Part model, mm, in its own coordinate system. A direction names the side the tool comes from. Round coordinates to 2 decimals unless told otherwise and drop trailing zeros. Order: outer loops, then holes, each group sorted by start corner. A loop starts at its lowest first (then second) coordinate and runs counter-clockwise, first axis right, second up. Notation, with made-up numbers: (47, 40) - (55, 40) arc R17 ccw to (55, 70) - close; hole circle Ø10 at (-8, -37.5). An arc over 180 degrees is marked (long way). Return JSON: item names as keys, results as strings. Group by question number.
Item 1: Two-plate mould, pull along X, no slides. Class faces 3 (the face through (8, 55, -2)), 4 (the face through (3, 6, -7)), 5 (the face through (15, 20, -3)): released by +X, released by -X, zero draft, split by the parting line, or undercut.
Item 2: Saw through at B-B on z = -9. List the corners of the cut face in (x, y), and give its area (3 significant figures).
Item 3: Saw through at C-C on y = 37. List the corners of the cut face in (x, z), and give its area (3 significant figures).
Item 4: Saw through at A-A on x = 7.5. List the corners of the cut face in (y, z).
Item 5: Drop flat-ended pins along their axis: pin 1 (1 mm diameter, centred on x = 11.5, y = 14.5, fed in from -Z); pin 2 (6 mm diameter, centred on x = 4, z = -11.5, fed in from +Y). Give the stop position or say it passes through.
Item 6: Probe probe 1 along Z at (x, y) = (13.25, 39); probe 2 along X at (y, z) = (2.35, -9); probe 3 along Y at (x, z) = (6.5, -6.5). List the from-to ranges inside material, lowest first.
Item 7: Tool access for faces 1 (the face through (5, 3, -11)), 2 (the face through (7, 1, -15)): list every direction of +Z, -Z, +X, -X, +Y, -Y with a clear straight run to the whole face (end or side of a thin tool).
Item 8: Saw through at D-D on x = 11.25. List the corners of the cut face in (y, z).
```python
from build123d import *

# Parameters (mm, degrees)
SKETCH1_W           = 15
SKETCH1_H           = 15
SKETCH1_R           = 2.65
BOSS_EXTRUDE1_DEPTH = 3
SKETCH2_W           = 15
SKETCH2_H           = 4
BOSS_EXTRUDE2_DEPTH = 54
BOSS_EXTRUDE3_DEPTH = 3
SKETCH4_R           = 1.65
CUT_EXTRUDE1_DEPTH  = 13
CUT_EXTRUDE2_DEPTH  = 20


with BuildPart() as part:
    # Sketch1 → Boss-Extrude1 (new body)
    with BuildSketch(Plane(origin=(0, 0, 0), x_dir=(1, 0, 0), z_dir=(0, 1, 0))):
        with Locations((7.5, 7.5)):
            Rectangle(SKETCH1_W, SKETCH1_H)
        with Locations(Location((7.5, 9, 0), (0, 0, 270))):
            Circle(SKETCH1_R, mode=Mode.SUBTRACT)
    extrude(amount=BOSS_EXTRUDE1_DEPTH)

    # Sketch2 → Boss-Extrude2 (add)
    with BuildSketch(Plane(origin=(0, 3, 0), x_dir=(1, 0, 0), z_dir=(0, 1, 0))):
        with Locations((7.5, 2)):
            Rectangle(SKETCH2_W, SKETCH2_H)
    extrude(amount=BOSS_EXTRUDE2_DEPTH)

    # Sketch3 → Boss-Extrude3 (add)
    with BuildSketch(Plane(origin=(15, 0, 0), x_dir=(0, 0, -1), z_dir=(1, 0, 0))):
        Polygon((4, 14), (15, 3), (4, 3), align=None)
    boss_extrude3 = extrude(amount=-BOSS_EXTRUDE3_DEPTH)

    # Mirror1: Boss-Extrude3 across plane
    add(boss_extrude3.mirror(Plane.ZY.offset(-7.5)))

    # Sketch4 → Cut-Extrude1 (cut)
    with BuildSketch(Plane(origin=(0, 0, -4), x_dir=(-1, 0, 0), z_dir=(0, 0, -1))):
        with Locations((-7.5, 37)):
            Circle(SKETCH4_R)
    extrude(amount=-CUT_EXTRUDE1_DEPTH, mode=Mode.SUBTRACT)

    # Sketch5 → Cut-Extrude2 (cut)
    with BuildSketch(Plane(origin=(15, 0, 0), x_dir=(0, 0, -1), z_dir=(1, 0, 0))):
        Polygon((0, 57), (4, 53), (4, 57), align=None)
    extrude(amount=-CUT_EXTRUDE2_DEPTH, mode=Mode.SUBTRACT)


solid = part.part
```
Filled in:
{
 "1": {"face 3": "zero draft", "face 4": "undercut", "face 5": "released by +X"},
 "2": {"outline": "(0, 0) - (4.85, 0) - (4.85, 3) - (3, 3) - (3, 9) - (0, 9) - close; (10.15, 0) - (15, 0) - (15, 9) - (12, 9) - (12, 3) - (10.15, 3) - close", "area": "65.1 mm^2"},
 "3": {"outline": "(0, -4) - (5.85, -4) - (5.85, 0) - (0, 0) - close; (9.15, -4) - (15, -4) - (15, 0) - (9.15, 0) - close", "area": "46.8 mm^2"},
 "4": {"outline": "(0, -15) - (3, -15) - (3, -11.65) - (0, -11.65) - close; (0, -6.35) - (3, -6.35) - (3, -4) - (35.35, -4) - (35.35, 0) - (0, 0) - close; (38.65, -4) - (53, -4) - (57, 0) - (38.65, 0) - close"},
 "5": {"pin 1": "stops at z = -4", "pin 2": "stops at y = 9.33"},
 "6": {"probe 1": "z = -4 to 0", "probe 2": "x = 0 to 4.85, 10.15 to 15", "probe 3": "y = 0 to 3"},
 "7": {"face 1": "-Z, +Y", "face 2": "-Z, +X, -X, +Y, -Y"},
 "8": {"outline": "(0, -15) - (3, -15) - (3, -4) - (53, -4) - (57, 0) - (0, 0) - close"}
}
